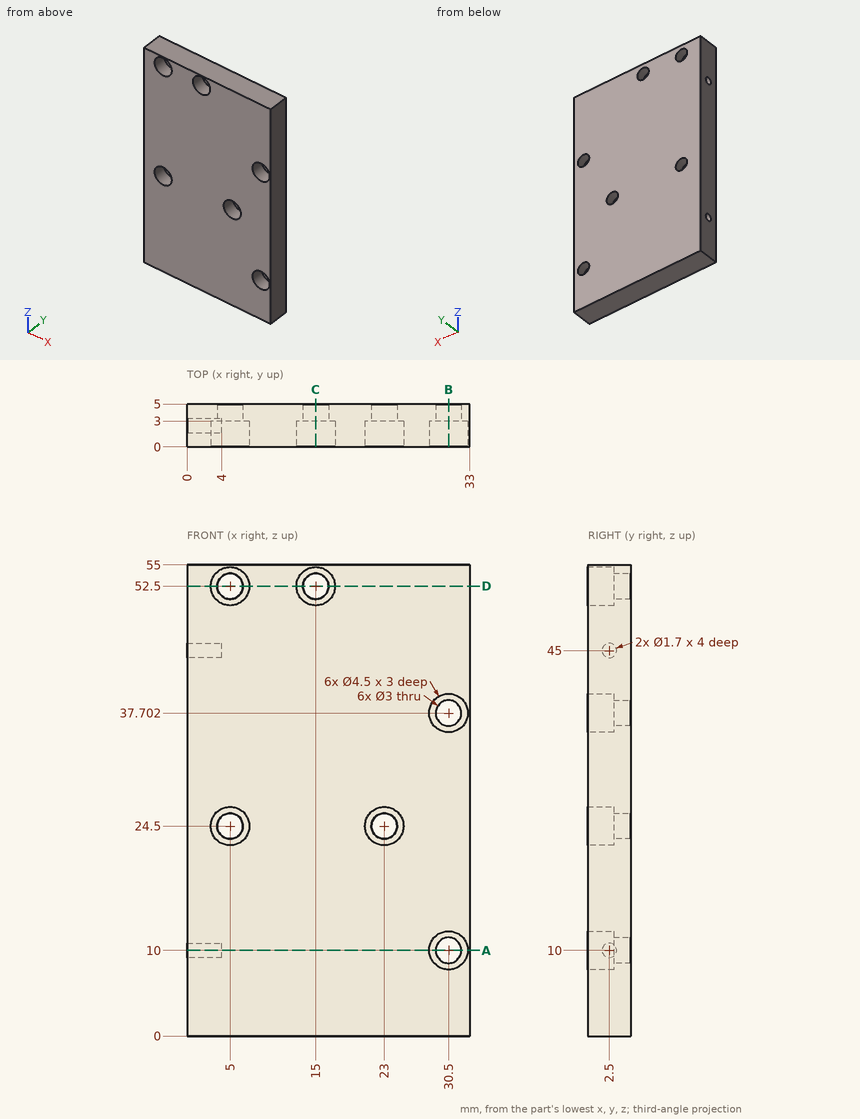
Design review of the part shown in the three views and the two pictorial views. Dimensions are in mm from the part's minimum x, y and z. Give positions to 0.01 mm unless a question says otherwise; leave off trailing zeros. Loops run counter-clockwise (first coordinate to the right, second up) from the corner with the lowest first, then second, coordinate; pieces in that order, holes last. Notation, with made-up numbers: (-30, -21.5) -> (-24, -21.5) arc R33 cw to (-24, 17.5) -> close; hole circle Ø8 at (56, 58). An arc over 180 degrees is marked (long way). One line per question, with ' | ' between items.
1) To check wall thickness, follow probe 1 along X at (y, z) = (2.3, 24.5); probe 2 along Z at (x, y) = (5, 4.35); probe 3 along X at (y, z) = (1.25, 26). State the ranges of each line that lie inside material, in increasing order.
Resolved:
probe 1: x = 0 to 2.75, 7.25 to 20.75, 25.25 to 33 | probe 2: z = 0 to 23, 26 to 51, 54 to 55 | probe 3: x = 0 to 3.32, 6.68 to 21.32, 24.68 to 33
2) Insertion check: pin 1 Ø1.3 at (x, z) = (5.5, 25.5) entering from -Y. The pin has a flat end and moves straight along its axis. Give the tip position at first contact, or say it passes through.
Resolved:
pin 1: stops at y = 3
3) We need section D-D (z = 52.5). Write out the cut boundary in (x, y), plus the area to 3 significant figures.
Resolved:
outline: (0, 0) -> (2.75, 0) -> (2.75, 3) -> (3.5, 3) -> (3.5, 5) -> (0, 5) -> close; (6.5, 3) -> (7.25, 3) -> (7.25, 0) -> (12.75, 0) -> (12.75, 3) -> (13.5, 3) -> (13.5, 5) -> (6.5, 5) -> close; (16.5, 3) -> (17.25, 3) -> (17.25, 0) -> (33, 0) -> (33, 5) -> (16.5, 5) -> close | area: 126 mm2
4) We need section A-A (z = 10). Write out the cut boundary in (x, y), plus the area to 3 significant figures.
Resolved:
outline: (0, 0) -> (28.25, 0) -> (28.25, 3) -> (29, 3) -> (29, 5) -> (0, 5) -> (0, 3.35) -> (4, 3.35) -> (4, 1.65) -> (0, 1.65) -> close; (32, 3) -> (32.75, 3) -> (32.75, 0) -> (33, 0) -> (33, 5) -> (32, 5) -> close | area: 139 mm2
5) We need section C-C (x = 15). Write out the cut boundary in (y, z), plus the area to 4 significant figures.
Resolved:
outline: (0, 0) -> (5, 0) -> (5, 51) -> (3, 51) -> (3, 50.25) -> (0, 50.25) -> close; (0, 54.75) -> (3, 54.75) -> (3, 54) -> (5, 54) -> (5, 55) -> (0, 55) -> close | area: 255.5 mm2
6) We need section B-B (x = 30.5). Write out the cut boundary in (y, z).
Resolved:
outline: (0, 0) -> (5, 0) -> (5, 8.5) -> (3, 8.5) -> (3, 7.75) -> (0, 7.75) -> close; (0, 12.25) -> (3, 12.25) -> (3, 11.5) -> (5, 11.5) -> (5, 36.2) -> (3, 36.2) -> (3, 35.45) -> (0, 35.45) -> close; (0, 39.95) -> (3, 39.95) -> (3, 39.2) -> (5, 39.2) -> (5, 55) -> (0, 55) -> close
